For this review, take the finished solid that the model builds, in its own axes (mm). A direction names the side the tool comes from. Round coordinates to 2 decimals unless told otherwise and drop trailing zeros. Write each loop counter-clockwise with the first axis right and the second up, starting at its lowest first coordinate (ties: lowest second). Pieces come first, ordered by that corner, then holes. Notation, with made-up numbers: (63.25, 41) -> (81.25, 41) arc R23 ccw to (81.25, 58) -> close; hole circle Ø9 at (36.5, 82). An arc over 180 degrees is marked (long way). Write each question's results on one line, items separated by ' | '. Start each with the question number.
Item 1: Clearance check with flat-ended pins moving along their axes: pin 1 (5 mm diameter, centred on x = -53.5, y = -25, fed in from -Z); pin 2 (1.3 mm diameter, centred on x = 169, z = 0, fed in from +Y); pin 3 (1.3 mm diameter, centred on x = 165.5, z = 0, fed in from -Y); pin 4 (6 mm diameter, centred on y = -59.5, z = 5.5, fed in from +X). State where each tip first meets the part, or that it passes through.
Item 2: Tool access review of faces 4 (the flat face through (-25, -101, 0.794)), 5 (the flat face through (-25, 101, -0.794)), 6 (the flat face through (134.47, 45.17, 0.01)), 7 (the flat face through (-25, -101, -0.794)), 8 (the flat face through (144, 0.794, 32)): name each direction out of +Z, -Z, +X, -X, +Y, -Y from which nothing blocks a thin tool from reaching the whole face with its end or side.
Item 3: Add section B-B (z = 22). State the section outline as (x, y) points, plus the area to 3 significant figures.
Item 4: To check wall thickness, follow line 1 along Z through (x, y) = (-39, -135.5); line 2 along X through (y, z) = (-3, -1); line 3 along Y through (x, z) = (19, 2.5). State the ranges of each line that lie inside material, in increasing order.
Item 5: Add section C-C (x = -126.5). State the section outline as (y, z) points.
Item 6: Add section A-A (y = 48). State the section outline as (x, z) points, plus the area to 3 significant figures.
Item 7: The part is to be moulded in two halves that separate along X. For faces 1 (the flat face through (-25, 101, 0.794)), 2 (the flat face through (134.47, -45.17, 0.01)), 3 (the flat face through (168.286, -42.004, 0.011)), say which applies: +X half, -X half, draft (parallel to the pull), parting line (faces both ways), or undercut.
from build123d import *

# Parameters (mm, degrees)
SKETCH1_W           = 318
SKETCH1_H           = 8
BOSS_EXTRUDE1_DEPTH = 4.8
SKETCH3_W           = 80
SKETCH3_H           = 195
BOSS_EXTRUDE2_DEPTH = 0.79375
BOSS_EXTRUDE3_DEPTH = 0.79375
BOSS_EXTRUDE4_DEPTH = 0.79375
FILLET1_R           = 2.5


with BuildPart() as part:
    # Sketch1 → Boss-Extrude1 (new, symmetric)
    with BuildSketch(Plane.XY):
        Rectangle(SKETCH1_W, SKETCH1_H)
    extrude(amount=BOSS_EXTRUDE1_DEPTH, both=True)

    # Sketch3 → Boss-Extrude2 (add, symmetric)
    with BuildSketch(Plane.XY):
        with Locations((-24, 97.5)):
            Rectangle(SKETCH3_W, SKETCH3_H)
    boss_extrude2 = extrude(amount=BOSS_EXTRUDE2_DEPTH, both=True)

    # Mirror1: Boss-Extrude2 across plane
    add(boss_extrude2.mirror(Plane.ZX))

    # Sketch6 → Boss-Extrude3 (add, symmetric)
    with BuildSketch(Plane(origin=(0, 0, 0), x_dir=(1, 0, 0), z_dir=(0, 1, 0))):
        Polygon((159, -4.8), (166.766007972, -74.8), (145.966007972, -74.8), (107, -4.8), align=None)
    extrude(amount=BOSS_EXTRUDE3_DEPTH, both=True)

    # Sketch8 → Boss-Extrude4 (add, symmetric)
    with BuildSketch(Plane.XY):
        Polygon((159, 0), (177.834948036, 85.2), (153.758948036, 85.2), (112.7, 0), align=None)
    boss_extrude4 = extrude(amount=BOSS_EXTRUDE4_DEPTH, both=True)

    # Mirror2: Boss-Extrude4 across plane
    add(boss_extrude4.mirror(Plane.ZX))

    # Fillet1
    fillet1_edges = [part.edges().sort_by_distance(p)[0] for p in [
        (-159, 0, 4.8),
        (-159, 0, -4.8),
    ]]
    fillet(fillet1_edges, radius=FILLET1_R)


solid = part.part
Responses:
1) pin 1: stops at z = -0.79 | pin 2: stops at y = 85.2 | pin 3: stops at y = -85.2 | pin 4: passes through
2) face 4: +Z, +X, -X, -Y | face 5: -Z, +X, -X, +Y | face 6: +Z, -Z, +Y | face 7: -Z, +X, -X, -Y | face 8: +Z, +X, -X, +Y
3) outline: (116.57, -0.79) -> (160.91, -0.79) -> (160.91, 0.79) -> (116.57, 0.79) -> close | area: 70.4 mm^2
4) line 1: z = -0.79 to 0.79 | line 2: x = -159 to 159 | line 3: y = -4 to 4
5) outline: (-4, -4.8) -> (4, -4.8) -> (4, 4.8) -> (-4, 4.8) -> close
6) outline: (-64, -0.79) -> (16, -0.79) -> (16, 0.79) -> (-64, 0.79) -> close; (135.83, -0.79) -> (169.61, -0.79) -> (169.61, 0.79) -> (135.83, 0.79) -> close | area: 181 mm^2
7) face 1: draft | face 2: undercut | face 3: +X half
